```python
from build123d import *

# Parameters (mm, degrees)
RIBCUT1_DEPTH    = 0.28575
RIBCUT2_DEPTH    = 0.4572
RIBCUTSPAT_COUNT = 12
RIBCUTSPAT_ANGLE = 330


with BuildPart() as part:
    # BodySke → BaseBody (revolve)
    with BuildSketch(Plane.XY):
        with BuildLine():
            Line((0, 0), (0, 2.77876))
            Line((0, 2.77876), (0.00508, 2.77876))
            Line((0.00508, 2.77876), (0.00508, 2.78384))
            ThreePointArc((0.00508, 2.78384), (0.23114, 3.0099), (0.4572, 2.78384))
            Line((0.4572, 2.78384), (0.4572, 2.7178))
            Line((0.4572, 2.7178), (0.9144, 2.4003))
            Line((0.9144, 2.4003), (0.9144, 2.0828))
            Line((0.9144, 2.0828), (9.05256, 2.0828))
            Line((9.05256, 2.0828), (9.525, 1.61036))
            Line((9.525, 1.61036), (9.525, 0))
            Line((9.525, 0), (0, 0))
        make_face()
    revolve(axis=Axis((0, 0, 0), (1, 0, 0)))

    # RibCut1Ske → RibCut1 (cut)
    with BuildSketch(Plane(origin=(0.9144, 0, 0), x_dir=(0, 0, -1), z_dir=(1, 0, 0))):
        with BuildLine():
            Line((0.271859953, 2.064981357), (0.271859953, 2.997597401))
            ThreePointArc((0.271859953, 2.997597401), (0.779019444, 2.907340145), (1.263361075, 2.731925476))
            Line((1.263361075, 2.731925476), (0.797053053, 1.92425629))
            ThreePointArc((0.797053053, 1.92425629), (0.539068307, 2.011830311), (0.271859953, 2.064981357))
        make_face()
    ribcut1 = extrude(amount=-RIBCUT1_DEPTH, mode=Mode.SUBTRACT)

    # RibCut2Ske → RibCut2 (cut)
    with BuildSketch(Plane(origin=(0.9144, 0, 0), x_dir=(0, 0, -1), z_dir=(1, 0, 0))):
        with BuildLine():
            Line((0.271859953, 2.384854766), (0.271859953, 2.997597401))
            ThreePointArc((0.271859953, 2.997597401), (0.779019444, 2.907340145), (1.263361075, 2.731925476))
            Line((1.263361075, 2.731925476), (0.956989757, 2.201274788))
            ThreePointArc((0.956989757, 2.201274788), (0.621243354, 2.318511761), (0.271859953, 2.384854766))
        make_face()
    ribcut2 = extrude(amount=-RIBCUT2_DEPTH, mode=Mode.SUBTRACT)

    # RibCutsPat: RibCut1, RibCut2 ×12 about axis
    ribcutspat_axis = Axis((0, 0, 0), (1, 0, 0))
    for i in range(1, RIBCUTSPAT_COUNT):
        add(ribcut1.rotate(ribcutspat_axis, i * RIBCUTSPAT_ANGLE / (RIBCUTSPAT_COUNT - 1)), mode=Mode.SUBTRACT)
        add(ribcut2.rotate(ribcutspat_axis, i * RIBCUTSPAT_ANGLE / (RIBCUTSPAT_COUNT - 1)), mode=Mode.SUBTRACT)


solid = part.part
```
Read the model definition and answer for the solid it produces. Units are mm, in the model's axes. Round coordinates to 2 decimals unless told otherwise and drop trailing zeros. Loops run counter-clockwise (first coordinate to the right, second up) from the corner with the lowest first, then second, coordinate; pieces in that order, holes last. Notation, with made-up numbers: (33.25, 60) -> (40.25, 60) arc R31 ccw to (40.25, 87) -> close; hole circle Ø4 at (67, -26.75). An arc over 180 degrees is marked (long way). One line per item, written item: value.
1) Consider L1, parallel to Z at x = 4.25, y = 0; L2, parallel to X at y = 2.75, z = -0.5; L3, parallel to Y at x = 1.5, z = 0.25. Determine where each line is inside the solid, lowest interval first. Write a range as [from, to].
Answer list:
L1: z = [-2.08, 2.08]
L2: x = [0.01, 0.46]
L3: y = [-2.07, 2.07]
2) A cutting plane is placed at C-C (x = 3.5). Determine the outline of the cut face in (y, z), and give its area (3 significant figures).
Answer list:
outline: circle Ø4.17 at (0, 0)
area: 13.6 mm²
3) Flat-ended cylindrical pins translate along their axes: P1, Ø0.5, axis at y = 1.5, z = -1.5, coming from the +X side; P2, Ø0.5, axis at x = 0.5, z = 2.5, coming from the +Y side; P3, Ø3, axis at x = 7.5, y = 1, coming from the -Z side. Find the tip coordinate at first contact, or state that the pin passes through.
Answer list:
P1: stops at x = 9.26
P2: stops at y = 1.89
P3: stops at z = -2.08
4) A cutting plane is placed at A-A (y = 0). Determine the outline of the cut face in (x, z) (3 decimals).
Answer list:
outline: (0, -2.779) -> (0.005, -2.779) -> (0.005, -2.784) arc R0.226 ccw to (0.457, -2.784) -> (0.457, -2.718) -> (0.914, -2.4) -> (0.914, -2.083) -> (9.053, -2.083) -> (9.525, -1.61) -> (9.525, 1.61) -> (9.053, 2.083) -> (0.914, 2.083) -> (0.914, 2.4) -> (0.457, 2.718) -> (0.457, 2.784) arc R0.226 ccw to (0.005, 2.784) -> (0.005, 2.779) -> (0, 2.779) -> close
